from build123d import *

# Parameters (mm, degrees)
F0_W          = 76.1676803231
F0_H          = 0.5
F0_W_2        = 68.4088433627
F0_H_2        = 3.77
F0_W_3        = 68.5331546701
F0_H_3        = 2.7
F0_H_4        = 2
F0_H_5        = 12
F1_DEPTH      = 50
F2_R          = 3
F3_DEPTH      = 70
F3_DEPTH_BACK = 0.501


with BuildPart() as f1:
    # F0 (on Front) → F1 (new body)
    with BuildSketch(Plane.XZ):
        Polygon((76.1676803231, 0), (0, 0), (0, -1.3), (2.9238497373, -1.3), (71.3326931, -1.3), (76.1956498027, -1.3), (76.1956498027, 0), align=None)
        Polygon((71.3326931, -60.04), (2.9238497373, -60.04), (0, -60.04), (0, -61.34), (76.1676803231, -61.34), (76.1956498027, -61.34), (76.1956498027, -60.04), align=None)
        Polygon((71.3326931, -5.07), (2.9238497373, -5.07), (0, -5.07), (0, -6.37), (2.8266510926, -6.37), (71.3598057628, -6.37), (76.290667057, -6.37), (76.290667057, -5.07), align=None)
        Polygon((71.3598057628, -8.37), (2.8266510926, -8.37), (0, -8.37), (0, -9.67), (2.8266510926, -9.67), (71.3598057628, -9.67), (76.290667057, -9.67), (76.290667057, -8.37), align=None)
        Polygon((71.3598057628, -51.67), (2.8266510926, -51.67), (0, -51.67), (0, -52.97), (2.8266510926, -52.97), (71.3598057628, -52.97), (76.290667057, -52.97), (76.290667057, -51.67), align=None)
        Polygon((71.3598057628, -12.37), (2.8266510926, -12.37), (0, -12.37), (0, -13.02), (2.8266510926, -13.02), (71.3598057628, -13.02), (76.290667057, -13.02), (76.290667057, -12.37), align=None)
        Polygon((71.3598057628, -25.02), (2.8266510926, -25.02), (0, -25.02), (0, -25.67), (2.8266510926, -25.67), (71.3598057628, -25.67), (76.290667057, -25.67), (76.290667057, -25.02), align=None)
        Polygon((71.3598057628, -54.97), (2.8266510926, -54.97), (0, -54.97), (0, -56.27), (2.9238497373, -56.27), (71.3326931, -56.27), (76.290667057, -56.27), (76.290667057, -54.97), align=None)
        Polygon((71.3598057628, -31.67), (2.8266510926, -31.67), (0, -31.67), (0, -32.97), (2.8266510926, -32.97), (71.3598057628, -32.97), (76.290667057, -32.97), (76.290667057, -31.67), align=None)
        Polygon((71.3598057628, -28.37), (2.8266510926, -28.37), (0, -28.37), (0, -29.67), (2.8266510926, -29.67), (71.3598057628, -29.67), (76.290667057, -29.67), (76.290667057, -28.37), align=None)
        with Locations((38.0838401616, 0.25)):
            Rectangle(F0_W, F0_H)
        with Locations((38.0838401616, -61.59)):
            Rectangle(F0_W, F0_H)
        Polygon((71.3598057628, -48.32), (2.8266510926, -48.32), (0, -48.32), (0, -48.97), (2.8266510926, -48.97), (71.3598057628, -48.97), (76.290667057, -48.97), (76.290667057, -48.32), align=None)
        Polygon((71.3598057628, -35.67), (2.8266510926, -35.67), (0, -35.67), (0, -36.32), (2.8266510926, -36.32), (71.3598057628, -36.32), (76.290667057, -36.32), (76.290667057, -35.67), align=None)
        with Locations((37.1282714186, -58.155)):
            Rectangle(F0_W_2, F0_H_2)
        with Locations((37.0932284277, -11.02)):
            Rectangle(F0_W_3, F0_H_3)
        with Locations((37.0932284277, -7.37)):
            Rectangle(F0_W_3, F0_H_4)
        with Locations((37.0932284277, -42.32)):
            Rectangle(F0_W_3, F0_H_5)
        with Locations((37.0932284277, -34.32)):
            Rectangle(F0_W_3, F0_H_3)
        with Locations((37.0932284277, -53.97)):
            Rectangle(F0_W_3, F0_H_4)
        with Locations((37.0932284277, -27.02)):
            Rectangle(F0_W_3, F0_H_3)
        with Locations((37.0932284277, -30.67)):
            Rectangle(F0_W_3, F0_H_4)
        with Locations((37.0932284277, -19.02)):
            Rectangle(F0_W_3, F0_H_5)
        with Locations((37.0932284277, -50.32)):
            Rectangle(F0_W_3, F0_H_3)
        with Locations((37.1282714186, -3.185)):
            Rectangle(F0_W_2, F0_H_2)
    extrude(amount=F1_DEPTH)

    # F2 (on Top) → F3 (cut, two sides)
    with BuildSketch(Plane.XY) as f3_sk:
        with Locations((0, -27.3095168173)):
            Circle(F2_R)
    extrude(amount=-F3_DEPTH, mode=Mode.SUBTRACT)
    extrude(f3_sk.sketch, amount=F3_DEPTH_BACK, mode=Mode.SUBTRACT)


solid = f1.part
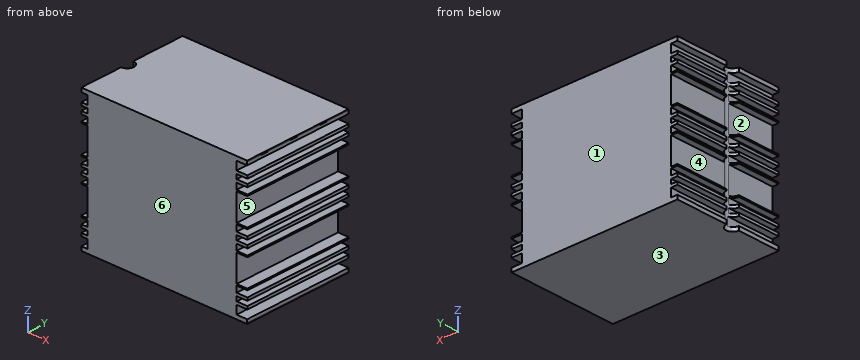
Work out the finished part from the listing and answer in its coordinate system (mm). Face numbers are marked on the shaded views. A direction names the side the tool comes from. Give positions to 0.01 mm unless a question says otherwise; leave off trailing zeros. Loops run counter-clockwise (first coordinate to the right, second up) from the corner with the lowest first, then second, coordinate; pieces in that order, holes last. Notation, with made-up numbers: (72.5, 55.25) -> (97.5, 55.25) arc R21 ccw to (97.5, 82.25) -> close; hole circle Ø2 at (31, 47.5). An arc over 180 degrees is marked (long way). Use a Markdown table: item, result. Add a question column.
1. For the marked faces 4, 5 and 6, determine the directions among +Z, -Z, +X, -X, +Y, -Y from which every point of the face is accessible in a straight line to the end or side of a thin tool.
2. Flat-ended cylindrical pins translate along their axes: pin 1 Ø6 at (x, z) = (25, -18) entering from +Y; pin 2 Ø1.9 at (y, z) = (-11, -57.5) entering from -X; pin 3 Ø1.4 at (y, z) = (-34, -27) entering from +X; pin 4 Ø6 at (y, z) = (-37, -43.5) entering from -X. Find the tip coordinate at first contact, or state that the pin passes through.
3. Determine the mould class of the marked faces 1, 2 and 3 for opening direction Z: released by +Z, released by -Z, zero draft, split by the parting line, or undercut.
4. Find the intervals of material crossed by probe 1 along X at (y, z) = (-4, -36.5); probe 2 along X at (y, z) = (-37.5, -3), in increasing order.
5. Section A-A on z = -15 is taken. Determine the outline of the cut face in (x, y).
Results below:
| question | item | result |
|---|---|---|
| 1 | face 4 | -X, +Y, -Y |
| 1 | face 5 | +X, +Y, -Y |
| 1 | face 6 | +Z, -Z, +X, -X, -Y |
| 2 | pin 1 | stops at y = 0 |
| 2 | pin 2 | stops at x = 2.92 |
| 2 | pin 3 | stops at x = 71.36 |
| 2 | pin 4 | stops at x = 2.83 |
| 3 | face 1 | zero draft |
| 3 | face 2 | undercut |
| 3 | face 3 | released by -Z |
| 4 | probe 1 | x = 2.83 to 71.36 |
| 4 | probe 2 | x = 2.92 to 71.33 |
| 5 | outline | (2.83, -50) -> (71.36, -50) -> (71.36, 0) -> (2.83, 0) -> (2.83, -26.3) arc R3 cw to (2.83, -28.31) -> close |
